from build123d import *

# Parameters (mm, degrees)
F0_R     = 30.25
F0_R_2   = 2
F1_DEPTH = 24
F0_R_3   = 1.25
F2_DEPTH = 23
F5_R     = 9.125
F5_R_2   = 8
F6_DEPTH = 25
F7_DEPTH = 15


# Not quite as in the source:
# - a fillet or chamfer that OpenCascade refuses, or shapes differently, is made with other operations: its cross-section is extruded or revolved along the edge and cut away or added


with BuildPart() as f1:
    # F0 (on Front) → F1 (new body)
    with BuildSketch(Plane.XZ):
        Circle(F0_R)
        with Locations((0, -20.07)):
            Circle(F0_R_2, mode=Mode.SUBTRACT)
        with Locations((18.6195461814, -10.75)):
            Circle(F0_R_2, mode=Mode.SUBTRACT)
        with BuildLine():
            ThreePointArc((-16.6195461814, 10.75), (-16.6876945288, 10.2323619098), (-16.8874953738, 9.75))
            ThreePointArc((-16.8874953738, 9.75), (-20.5513978339, 11.2676380902), (-16.6195461814, 10.75))
        make_face(mode=Mode.SUBTRACT)
        with BuildLine():
            ThreePointArc((8.875, 15.3719509172), (14.3703479176, 10.4190019065), (17.369375, 3.6561334917))
            ThreePointArc((17.369375, 3.6561334917), (23.9351114309, 5.5736293158), (27.9, 0))
            ThreePointArc((27.9, 0), (23.9351114309, -5.5736293158), (17.369375, -3.6561334917))
            ThreePointArc((17.369375, -3.6561334917), (0, -17.75), (-17.369375, -3.6561334917))
            ThreePointArc((-17.369375, -3.6561334917), (-27.9, 0), (-17.369375, 3.6561334917))
            ThreePointArc((-17.369375, 3.6561334917), (-16.5773263107, 6.3446632999), (-15.3719509172, 8.875))
            ThreePointArc((-15.3719509172, 8.875), (-4.5940380506, 17.1451834166), (8.875, 15.3719509172))
        make_face(mode=Mode.SUBTRACT)
        with Locations((0, 20.07)):
            Circle(F0_R_2, mode=Mode.SUBTRACT)
    extrude(amount=F1_DEPTH)

    # F0 (on Front) → F2 (join)
    with BuildSketch(Plane.XZ):
        with BuildLine():
            ThreePointArc((-17.369375, 3.6561334917), (-27.9, 0), (-17.369375, -3.6561334917))
            ThreePointArc((-17.369375, -3.6561334917), (-17.75, 0), (-17.369375, 3.6561334917))
        make_face()
        with Locations((-22, 0)):
            Circle(F0_R_3, mode=Mode.SUBTRACT)
        with Locations((0, 20.07)):
            Circle(F0_R_2)
        with BuildLine():
            ThreePointArc((17.369375, 3.6561334917), (17.6545873111, 1.8379463744), (17.75, 0))
            ThreePointArc((17.75, 0), (17.6545873111, -1.8379463744), (17.369375, -3.6561334917))
            ThreePointArc((17.369375, -3.6561334917), (23.9351114309, -5.5736293158), (27.9, 0))
            ThreePointArc((27.9, 0), (23.9351114309, 5.5736293158), (17.369375, 3.6561334917))
        make_face()
        with Locations((22, 0)):
            Circle(F0_R_3, mode=Mode.SUBTRACT)
        with Locations((0, -20.07)):
            Circle(F0_R_2)
    extrude(amount=F2_DEPTH)

    # F3: chamfer of 3 on 2 edges, made by hand

    # F3_s1 → F3_t2 (revolve, cut)
    with BuildSketch(Plane.XY.offset(10.75)):
        Polygon((-13.6195461814, -24), (-16.6195461814, -21), (-16.6195461814, -24), align=None)
    revolve(axis=Axis((-18.6195461814, -24, 10.75), (0, -1, 0)), mode=Mode.SUBTRACT)

    # F3_s3 → F3_t4 (revolve, cut)
    with BuildSketch(Plane.XY.offset(-10.75)):
        Polygon((23.6195461814, -24), (20.6195461814, -21), (20.6195461814, -24), align=None)
    revolve(axis=Axis((18.6195461814, -24, -10.75), (0, -1, 0)), mode=Mode.SUBTRACT)

    # F5 (on offset) → F6 (cut)
    with BuildSketch(Plane.XY.offset(18.75)):
        with Locations((0, -12.125)):
            Circle(F5_R)
        with Locations((0, -12.125)):
            Circle(F5_R_2, mode=Mode.SUBTRACT)
    extrude(amount=F6_DEPTH, mode=Mode.SUBTRACT)

    # F5 (on offset) → F7 (cut, symmetric)
    with BuildSketch(Plane.XY.offset(18.75)):
        with Locations((0, -12.125)):
            Circle(F5_R_2)
    extrude(amount=F7_DEPTH, both=True, mode=Mode.SUBTRACT)


solid = f1.part
Source: CAD feature listing. Evaluate the final solid. Frame: model axes, mm. A direction names the side the tool comes from. Round coordinates to 2 decimals unless told otherwise and drop trailing zeros. Loops run counter-clockwise (first coordinate to the right, second up) from the corner with the lowest first, then second, coordinate; pieces in that order, holes last. Notation, with made-up numbers: M 5,-26.75 L 33,-26.75 A4 ccw 33,-20.75 Z; hole C 41,40 d2. An arc over 180 degrees is marked long. Return JSON: item names as keys, results as strings. Group by question number.
1. Section query C-C on z = -19. Output: boundary loops of the cut face in (x, y).
2. Reachability of faces 1 (the face through (0, -23, -20)), 2 (the face through (23.155, -11.339, -0.479)), 3 (the face through (3, -20, 18.75)) from +Z, -Z, +X, -X, +Y, -Y: full face, straight path, thin tool, end or side. Return the list, or none.
3. Mould query, pull axis Z, two halves, no side actions, for faces 4 (the face through (13, -24, -13)), 5 (the face through (-23, -23, -1)), 6 (the face through (-6.56, -11.83, -29.53)). Classes: released by +Z, released by -Z, zero draft, split by the parting line, or undercut.
4. Pin query (flat end, axial travel): pin 1 (3 mm diameter, centred on x = 24.5, z = 0, fed in from -Y); pin 2 (13 mm diameter, centred on x = 0, y = -12.125, fed in from -Z); pin 3 (2 mm diameter, centred on x = -22, z = 0, fed in from -Y); pin 4 (9 mm diameter, centred on x = 1, y = -14.5, fed in from +Z). Return the tip coordinate at first contact, or that it passes through.
5. Section query B-B on y = -5.5. State how many separate pieces and enclosed holes the cut face has, and give its area (3 significant figures).
6. Material intervals for line 1 along Z through (x, y) = (0, -23.5); line 2 along Y through (x, z) = (0, 24); line 3 along X through (y, z) = (-22.25, 9.5), sorted ascending. Write a range as from..to.
7. Section query A-A on z = 20.07. Output: boundary loops of the cut face in (x, y) (3 decimals).
Checks:
{
 "1": {"outline": "M -23.54,-24 L -1.69,-24 L -1.69,-23 L 1.69,-23 L 1.69,-24 L 23.54,-24 L 23.54,0 L -23.54,0 Z"},
 "2": {"face 1": "-Y", "face 2": "+Y, -Y", "face 3": "+Z"},
 "3": {"face 4": "zero draft", "face 5": "undercut", "face 6": "split by the parting line"},
 "4": {"pin 1": "stops at y = -23", "pin 2": "stops at z = -30.25", "pin 3": "passes through", "pin 4": "stops at z = -16.88"},
 "5": {"separate pieces": "1", "enclosed holes": "4", "area": "1,700 mm²"},
 "6": {"line 1": "z = -30.25..-22.07, -18.07..-17.75, 17.75..18.07, 22.07..30.25", "line 2": "y = -24..-21.25, -3..0", "line 3": "x = -28.72..-21.62, -15.62..-14.99, 14.99..28.72"},
 "7": {"outline": "M -22.633,-24 L -2,-24 L -2,-23 L 2,-23 L 2,-24 L 22.633,-24 L 22.633,0 L -22.633,0 Z; hole C 0,-12.125 d18.25"}
}
